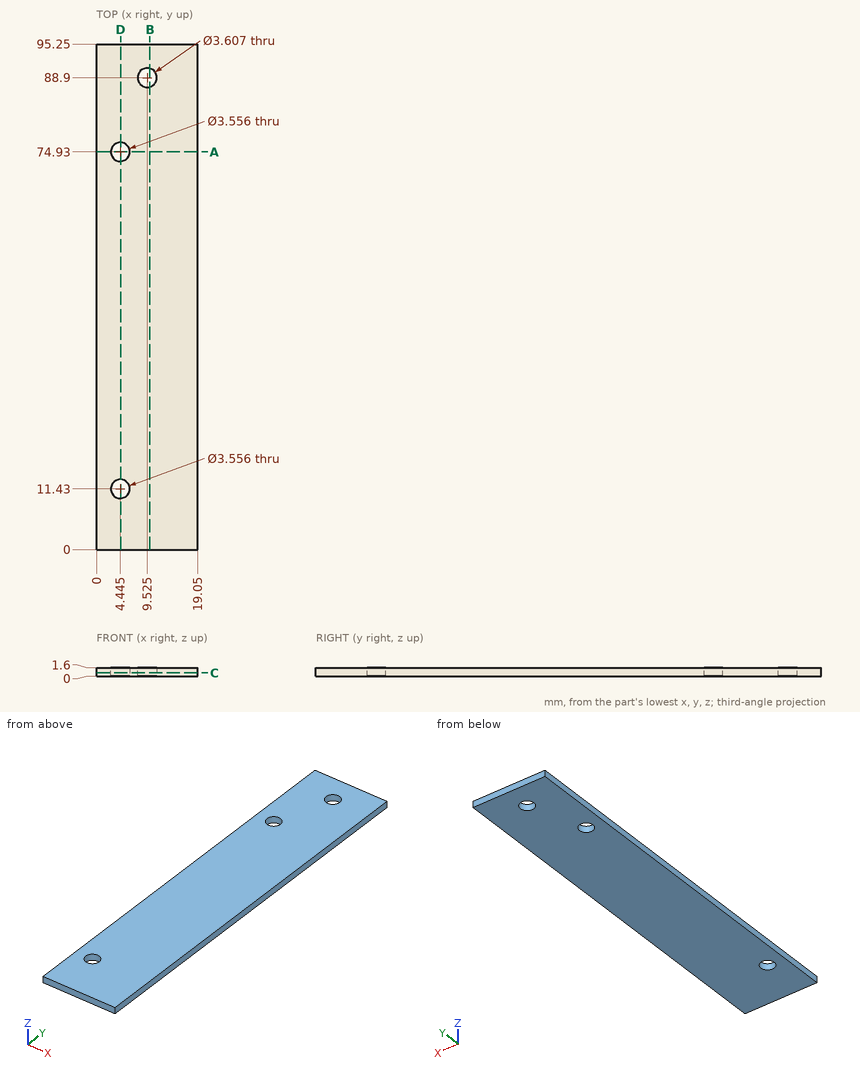
Source: three-view drawing plus pictorial views. Frame: mm from the lowest corner of the part. Give positions to 0.01 mm unless a question says otherwise; leave off trailing zeros. Write each loop counter-clockwise with the first axis right and the second up, starting at its lowest first coordinate (ties: lowest second). Pieces come first, ordered by that corner, then holes.
(1) Cut plane C-C, the plane z = 0.6. Give the number of separate pieces and of enclosed holes in the cut face, then the cut area to 3 significant figures.
(2) Ray query, line 1 (X direction, y = 74.93, z = 0.7); line 2 (Y direction, x = 5.5, z = 1.4); line 3 (Y direction, x = 5.75, z = 0.5). Return the intervals inside material, ascending.
(3) Cut plane D-D, the plane x = 4.5. Return loops of the section in (y, z).
(4) Cut plane A-A, the plane y = 74.93. Return loops of the section in (x, z).
(5) Cut plane B-B, the plane x = 10. Return loops of the section in (y, z).
Values follow:
1. separate pieces: 1
1. enclosed holes: 3
1. area: 1,780 mm2
2. line 1: x = 0 to 2.67, 6.22 to 19.05
2. line 2: y = 0 to 10, 12.86 to 73.5, 76.36 to 95.25
2. line 3: y = 0 to 10.22, 12.64 to 73.72, 76.14 to 95.25
3. outline: (0, 0) - (9.65, 0) - (9.65, 1.6) - (0, 1.6) - close; (13.21, 0) - (73.15, 0) - (73.15, 1.6) - (13.21, 1.6) - close; (76.71, 0) - (95.25, 0) - (95.25, 1.6) - (76.71, 1.6) - close
4. outline: (0, 0) - (2.67, 0) - (2.67, 1.6) - (0, 1.6) - close; (6.22, 0) - (19.05, 0) - (19.05, 1.6) - (6.22, 1.6) - close
5. outline: (0, 0) - (87.16, 0) - (87.16, 1.6) - (0, 1.6) - close; (90.64, 0) - (95.25, 0) - (95.25, 1.6) - (90.64, 1.6) - close
